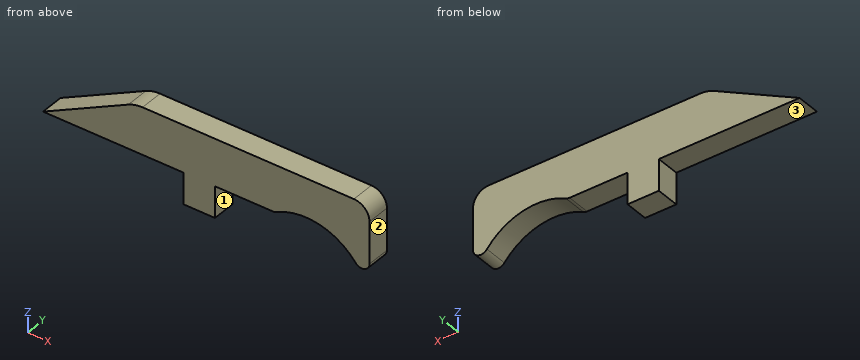
```python
from build123d import *

# Parameters (mm, degrees)
BOSS_EXTRUDE1_DEPTH = 4.7625
FILLET1_R           = 1.5875
FILLET2_R           = 6.35
FILLET3_R           = 3.175
SKETCH6_W           = 6.35
SKETCH6_H           = 4.7625
BOSS_EXTRUDE2_DEPTH = 6.35


with BuildPart() as part:
    # Sketch1 → Boss-Extrude1 (new body)
    with BuildSketch(Plane(origin=(0, 0, 0), x_dir=(1, 0, 0), z_dir=(0, 1, 0))):
        with BuildLine():
            ThreePointArc((71.8451, -2.691968416), (65.44608311, -13.792101845), (52.633598926, -13.817168416))
            Line((52.633598926, -13.817168416), (5.5225, -13.817168416))
            Line((5.5225, -13.817168416), (24.2201, -23.342168416))
            Line((24.2201, -23.342168416), (71.8451, -23.342168416))
            Line((71.8451, -23.342168416), (71.8451, -2.691968416))
        make_face()
    extrude(amount=BOSS_EXTRUDE1_DEPTH)

    # Fillet1
    fillet1_edges = [part.edges().sort_by_distance(p)[0] for p in [
        (71.8451, 2.38125, 2.691968416),
        (52.633598926, 2.38125, 13.817168416),
    ]]
    fillet(fillet1_edges, radius=FILLET1_R)

    # Fillet2
    fillet2_edges = [part.edges().sort_by_distance(p)[0] for p in [
        (24.2201, 2.38125, 23.342168416),
    ]]
    fillet(fillet2_edges, radius=FILLET2_R)

    # Fillet3
    fillet3_edges = [part.edges().sort_by_distance(p)[0] for p in [
        (71.8451, 2.38125, 23.342168416),
    ]]
    fillet(fillet3_edges, radius=FILLET3_R)

    # Sketch6 → Boss-Extrude2 (add)
    with BuildSketch(Plane(origin=(0, 0, 13.817168416), x_dir=(-1, 0, 0), z_dir=(0, 0, -1))):
        with Locations((-37.2725, 2.38125)):
            Rectangle(SKETCH6_W, SKETCH6_H)
    extrude(amount=BOSS_EXTRUDE2_DEPTH)


solid = part.part
```
Build history of the part. All positions in model axes, mm. Face numbers are marked on the shaded views. A direction names the side the tool comes from. Round coordinates to 2 decimals unless told otherwise and drop trailing zeros. Order: outer loops, then holes, each group sorted by start corner. A loop starts at its lowest first (then second) coordinate and runs counter-clockwise, first axis right, second up. Notation, with made-up numbers: (87.5, 83) -> (146.5, 83) arc R16 cw to (146.5, 93) -> close; hole circle Ø5 at (9, 63.5). An arc over 180 degrees is marked (long way). Answer in a Markdown table with one row per item.
1) Wall check: L1, parallel to X at y = 0.45, z = 9.25; L2, parallel to X at y = 0.2, z = 12; L3, parallel to Z at x = 31.5, y = 0.95. Give the ranges that are in metal, low to high.
Values:
| item | result |
|---|---|
| L1 | 34.1 to 40.45 |
| L2 | 34.1 to 40.45, 67.84 to 71.85 |
| L3 | 13.82 to 23.34 |
2) Pin check, flat tips, straight feed: P1, Ø2.5, axis at y = 1.5, z = 9.5, coming from the -X side; P2, Ø2, axis at x = 20, y = 0.5, coming from the +Z side; P3, Ø1.4, axis at x = 46.5, y = 3, coming from the -Z side. Stop position of each tip, or through.
Values:
| item | result |
|---|---|
| P1 | x = 34.1 |
| P2 | z = 21.7 |
| P3 | z = 13.82 |
3) Band-saw the part on A-A on z = 9. Give the cut face in (x, y).
Values:
| item | result |
|---|---|
| outline | (34.1, 0) -> (40.45, 0) -> (40.45, 4.76) -> (34.1, 4.76) -> close |
4) Which spindle directions (+Z, -Z, +X, -X, +Y, -Y) get a long thin tool onto all of the face, cutting with end or side? Do the marked faces 1, 2 and 3. Say none if no direction does.
Values:
| item | result |
|---|---|
| face 1 | -Z, +Y, -Y |
| face 2 | +Z, -Z, +X, +Y, -Y |
| face 3 | -Z, -X, +Y, -Y |
5) Band-saw the part on B-B on x = 45. Give the cut face in (y, z).
Values:
| item | result |
|---|---|
| outline | (0, 13.82) -> (4.76, 13.82) -> (4.76, 23.34) -> (0, 23.34) -> close |
